The listing builds one solid part. Answer for the finished solid, in the listing's coordinates (mm). A direction names the side the tool comes from. Round coordinates to 2 decimals unless told otherwise and drop trailing zeros. Order: outer loops, then holes, each group sorted by start corner. A loop starts at its lowest first (then second) coordinate and runs counter-clockwise, first axis right, second up. Notation, with made-up numbers: (37.25, 79) -> (63.25, 79) arc R31 cw to (63.25, 104) -> close; hole circle Ø2 at (2.5, 54.25). An arc over 180 degrees is marked (long way). Answer in a Markdown table with one row per item. Add a question column.
```python
from build123d import *

# Parameters (mm, degrees)
P_IDAT_VYSUNUT_M1_DEPTH = 7


with BuildPart() as part:
    # Skica1 → Přidat vysunutím1 (new body)
    with BuildSketch(Plane.XY):
        with BuildLine():
            Line((-11, 31.128764833), (-11, 70))
            Line((-11, 70), (-5.920908656, 100.97099984))
            ThreePointArc((-5.920908656, 100.97099984), (0, 106), (5.920908656, 100.97099984))
            Line((5.920908656, 100.97099984), (11, 70))
            Line((11, 70), (11, 31.128764833))
            ThreePointArc((11, 31.128764833), (11.732180215, 28.523824471), (13.714285714, 26.681798428))
            ThreePointArc((13.714285714, 26.681798428), (25.980762114, 15), (29.964258114, -1.463979391))
            ThreePointArc((29.964258114, -1.463979391), (30.568446713, -4.101546127), (32.458301133, -6.038102975))
            Line((32.458301133, -6.038102975), (66.121778265, -25.473720558))
            Line((66.121778265, -25.473720558), (90.403905235, -45.357842611))
            ThreePointArc((90.403905235, -45.357842611), (91.798692801, -53), (84.482996579, -55.61315723))
            Line((84.482996579, -55.61315723), (55.121778265, -44.526279442))
            Line((55.121778265, -44.526279442), (21.458301133, -25.090661858))
            ThreePointArc((21.458301133, -25.090661858), (18.836266498, -24.422278344), (16.2499724, -25.217819037))
            ThreePointArc((16.2499724, -25.217819037), (0, -30), (-16.2499724, -25.217819037))
            ThreePointArc((-16.2499724, -25.217819037), (-18.836266498, -24.422278344), (-21.458301133, -25.090661858))
            Line((-21.458301133, -25.090661858), (-55.121778265, -44.526279442))
            Line((-55.121778265, -44.526279442), (-84.482996579, -55.61315723))
            ThreePointArc((-84.482996579, -55.61315723), (-91.798692801, -53), (-90.403905235, -45.357842611))
            Line((-90.403905235, -45.357842611), (-66.121778265, -25.473720558))
            Line((-66.121778265, -25.473720558), (-32.458301133, -6.038102975))
            ThreePointArc((-32.458301133, -6.038102975), (-30.568446713, -4.101546127), (-29.964258114, -1.463979391))
            ThreePointArc((-29.964258114, -1.463979391), (-25.980762114, 15), (-13.714285714, 26.681798428))
            ThreePointArc((-13.714285714, 26.681798428), (-11.732180215, 28.523824471), (-11, 31.128764833))
        make_face()
        with BuildLine():
            Line((-5, 65), (-5, 40))
            ThreePointArc((-5, 40), (0, 35), (5, 40))
            Line((5, 40), (5, 65))
            ThreePointArc((5, 65), (0, 70), (-5, 65))
        make_face(mode=Mode.SUBTRACT)
        with BuildLine():
            Line((58.791651246, -28.169872981), (37.141016151, -15.669872981))
            ThreePointArc((37.141016151, -15.669872981), (30.310889132, -17.5), (32.141016151, -24.330127019))
            Line((32.141016151, -24.330127019), (53.791651246, -36.830127019))
            ThreePointArc((53.791651246, -36.830127019), (60.621778265, -35), (58.791651246, -28.169872981))
        make_face(mode=Mode.SUBTRACT)
        Polygon((0, -13.856406461), (12, -6.92820323), (12, 6.92820323), (0, 13.856406461), (-12, 6.92820323), (-12, -6.92820323), align=None, mode=Mode.SUBTRACT)
        with BuildLine():
            Line((-53.791651246, -36.830127019), (-32.141016151, -24.330127019))
            ThreePointArc((-32.141016151, -24.330127019), (-30.310889132, -17.5), (-37.141016151, -15.669872981))
            Line((-37.141016151, -15.669872981), (-58.791651246, -28.169872981))
            ThreePointArc((-58.791651246, -28.169872981), (-60.621778265, -35), (-53.791651246, -36.830127019))
        make_face(mode=Mode.SUBTRACT)
    extrude(amount=P_IDAT_VYSUNUT_M1_DEPTH)


solid = part.part
```
1. For faces 5 (the flat face through (-69.597, -49.992, 3.451)), 6 (the flat face through (49.054, -15.62, 3.451)), 7 (the flat face through (-12, 0, 3)), determine the directions among +Z, -Z, +X, -X, +Y, -Y from which every point of the face is accessible in a straight line to the end or side of a thin tool.
2. The part is cut by section C-C (z = 4.25). Give the number of separate pieces and of enclosed holes in the cut face, then the cut area to 3 significant figures.
3. The part is cut by section D-D (x = 68.5). Give the vertices of the cut face in (y, z), then the cut area to 3 significant figures.
4. The mould has two halves that part along Y. Classify faces 1 (the cylindrical face through (60.57, -35.09, 3.45)), 2 (the flat face through (38.526, -34.945, 3.451)), 3 (the flat face through (-11, 50, 3)), 4 (the flat face through (12, 0, 3)): released by +Y, released by -Y, zero draft, split by the parting line, or undercut.
5. Straight lines are drawn through the part: line 1 along X through (y, z) = (-16.5, 3); line 2 along Y through (x, z) = (-4.5, 5.5); line 3 along X through (y, z) = (54.5, 1.5). For each, find the intervals that lie inside material, in ascending order.
6. Each of these flat-tipped pins is pushed along its axis until it touches: pin 1 (2 mm diameter, centred on y = 50, z = 2.5, fed in from -X); pin 2 (4 mm diameter, centred on x = 13, z = 5.5, fed in from -Y); pin 3 (12 mm diameter, centred on x = 71, y = -27, fed in from -Z); pin 4 (4 mm diameter, centred on x = -27, z = 5, fed in from +Y). Where does it stop, or does it pass through?
7. The part is cut by section A-A (y = -32.5). Give the vertices of the cut face in (x, z), then the cut area to 3 significant figures.
8. The part is cut by section B-B (x = -9). Give the vertices of the cut face in (y, z).
Report:
| question | item | result |
|---|---|---|
| 1 | face 5 | +Z, -Z, -Y |
| 1 | face 6 | +Z, -Z, +X, +Y |
| 1 | face 7 | +Z, -Z |
| 2 | separate pieces | 1 |
| 2 | enclosed holes | 4 |
| 2 | area | 5,750 mm^2 |
| 3 | outline | (-49.58, 0) -> (-27.42, 0) -> (-27.42, 7) -> (-49.58, 7) -> close |
| 3 | area | 155 mm^2 |
| 4 | face 1 | undercut |
| 4 | face 2 | released by -Y |
| 4 | face 3 | zero draft |
| 4 | face 4 | undercut |
| 5 | line 1 | x = -50.58 to -38.58, -31.07 to 31.07, 38.58 to 50.58 |
| 5 | line 2 | y = -29.66 to -11.26, 11.26 to 37.82, 67.18 to 103.97 |
| 5 | line 3 | x = -11 to -5, 5 to 11 |
| 6 | pin 1 | stops at x = -11 |
| 6 | pin 2 | stops at y = -27.91 |
| 6 | pin 3 | stops at z = 0 |
| 6 | pin 4 | stops at y = 16.58 |
| 7 | outline | (-74.7, 0) -> (-61.29, 0) -> (-61.29, 7) -> (-74.7, 7) -> close; (-46.29, 0) -> (-34.29, 0) -> (-34.29, 7) -> (-46.29, 7) -> close; (34.29, 0) -> (46.29, 0) -> (46.29, 7) -> (34.29, 7) -> close; (61.29, 0) -> (74.7, 0) -> (74.7, 7) -> (61.29, 7) -> close |
| 7 | area | 356 mm^2 |
| 8 | outline | (-28.62, 0) -> (-8.66, 0) -> (-8.66, 7) -> (-28.62, 7) -> close; (8.66, 0) -> (82.2, 0) -> (82.2, 7) -> (8.66, 7) -> close |
